The listing builds one solid part. Answer for the finished solid, in the listing's coordinates (mm). A direction names the side the tool comes from. Coordinates: 2 decimals unless noted, no trailing zeros. Order: outer loops, then holes, each group sorted by start corner. A loop starts at its lowest first (then second) coordinate and runs counter-clockwise, first axis right, second up. Notation, with made-up numbers: (30.25, -35.5) -> (58.25, -35.5) arc R17 ccw to (58.25, -7.5) -> close; hole circle Ø6 at (-40, 23.25). An arc over 180 degrees is marked (long way). Return JSON: item names as keys, results as strings.
from build123d import *

# Parameters (mm, degrees)
ENL_V_MAT_EXTRU_1_DEPTH = 149.219431924
ESQUISSE3_R             = 3.75
ENL_V_MAT_EXTRU_2_DEPTH = 131.858702424
ENL_V_MAT_EXTRU_3_DEPTH = 126.862394907
ENL_V_MAT_EXTRU_4_DEPTH = 10
CONG_1_R                = 1


with BuildPart() as part:
    # Esquisse1 → Révolution1 (revolve)
    with BuildSketch(Plane.XY, mode=Mode.PRIVATE) as r_volution1_sk:
        with BuildLine():
            Line((0, 0), (24.566275292, 0))
            Line((24.566275292, 0), (24.566275292, 25))
            Line((24.566275292, 25), (7.566275292, 25))
            ThreePointArc((7.566275292, 25), (6.152061729, 25.585786438), (5.566275292, 27))
            Line((5.566275292, 27), (5.566275292, 40))
            Line((5.566275292, 40), (-22.933724708, 40))
            Line((-22.933724708, 40), (-25.433724708, 37.5))
            Line((-25.433724708, 37.5), (-62.433724708, 37.5))
            Line((-62.433724708, 37.5), (-64.933724708, 40))
            Line((-64.933724708, 40), (-93.433724708, 40))
            Line((-93.433724708, 40), (-93.433724708, 27))
            ThreePointArc((-93.433724708, 27), (-94.019511146, 25.585786438), (-95.433724708, 25))
            Line((-95.433724708, 25), (-112.433724708, 25))
            Line((-112.433724708, 25), (-112.433724708, 0))
            Line((-112.433724708, 0), (0, 0))
        make_face()
    revolve(r_volution1_sk.sketch.rotate(Axis((-130.768922499, 0, 0), (1, 0, 0)), 90), axis=Axis((-130.768922499, 0, 0), (1, 0, 0)))

    # Esquisse2 → Enlèv. mat.-Extru.1 (cut, through all)
    with BuildSketch(Plane.ZY.offset(112.433724708)):
        with BuildLine():
            Line((0, 7), (0, 0))
            Line((0, 0), (43.449782835, 0))
            Line((43.449782835, 0), (43.449782835, 44.497429883))
            Line((43.449782835, 44.497429883), (0, 44.497429883))
            Line((0, 44.497429883), (0, 13))
            ThreePointArc((0, 13), (3, 10), (0, 7))
        make_face()
        with BuildLine():
            Line((-12, 7), (0, 7))
            ThreePointArc((0, 7), (3, 10), (0, 13))
            Line((0, 13), (-12, 13))
            ThreePointArc((-12, 13), (-15, 10), (-12, 7))
        make_face()
    extrude(amount=-ENL_V_MAT_EXTRU_1_DEPTH, mode=Mode.SUBTRACT)

    # Esquisse3 → Enlèv. mat.-Extru.2 (cut, through all)
    with BuildSketch(Plane.ZY.offset(93.433724708)):
        with Locations((-8.282209443, 30.909626441)):
            Circle(ESQUISSE3_R)
        with Locations((-22.627416998, 22.627416998)):
            Circle(ESQUISSE3_R)
        with Locations((-30.909626441, 8.282209443)):
            Circle(ESQUISSE3_R)
        with Locations((-30.909626441, -8.282209443)):
            Circle(ESQUISSE3_R)
        with Locations((-22.627416998, -22.627416998)):
            Circle(ESQUISSE3_R)
        with Locations((-8.282209443, -30.909626441)):
            Circle(ESQUISSE3_R)
        with Locations((8.282209443, -30.909626441)):
            Circle(ESQUISSE3_R)
        with Locations((22.627416998, -22.627416998)):
            Circle(ESQUISSE3_R)
        with Locations((30.909626441, -8.282209443)):
            Circle(ESQUISSE3_R)
    extrude(amount=-ENL_V_MAT_EXTRU_2_DEPTH, mode=Mode.SUBTRACT)

    # Esquisse4 → Enlèv. mat.-Extru.3 (cut, through all)
    with BuildSketch(Plane(origin=(0, 0, 0), x_dir=(1, 0, 0), z_dir=(0, 1, 0))):
        with BuildLine():
            Line((5.566275292, -31.140154495), (24.566275292, -40))
            Line((24.566275292, -40), (21.921370581, -25))
            Line((21.921370581, -25), (7.566275292, -25))
            ThreePointArc((7.566275292, -25), (6.152061729, -25.585786438), (5.566275292, -27))
            Line((5.566275292, -27), (5.566275292, -31.140154495))
        make_face()
        with BuildLine():
            Line((-5.433724708, -40), (5.566275292, -40))
            Line((5.566275292, -40), (5.566275292, -31.140154495))
            Line((5.566275292, -31.140154495), (-2.622958319, -27.321452148))
            ThreePointArc((-2.622958319, -27.321452148), (-4.722604922, -33.506811582), (-5.433724708, -40))
        make_face()
        with BuildLine():
            Line((-2.622958319, -27.321452148), (5.566275292, -31.140154495))
            Line((5.566275292, -31.140154495), (5.566275292, -27))
            ThreePointArc((5.566275292, -27), (6.152061729, -25.585786438), (7.566275292, -25))
            Line((7.566275292, -25), (21.921370581, -25))
            Line((21.921370581, -25), (19.356829962, -10.45576741))
            ThreePointArc((19.356829962, -10.45576741), (6.303432421, -16.199399791), (-2.622958319, -27.321452148))
        make_face()
        Polygon((5.566275292, -40), (24.566275292, -40), (5.566275292, -31.140154495), align=None)
        with BuildLine():
            Line((-7.154497255, -25.208360839), (-2.622958319, -27.321452148))
            ThreePointArc((-2.622958319, -27.321452148), (6.303432421, -16.199399791), (19.356829962, -10.45576741))
            Line((19.356829962, -10.45576741), (18.488589073, -5.531728645))
            ThreePointArc((18.488589073, -5.531728645), (3.259625276, -12.23263309), (-7.154497255, -25.208360839))
        make_face()
        with BuildLine():
            Line((21.921370581, -25), (24.566275292, -25))
            Line((24.566275292, -25), (24.566275292, -10))
            ThreePointArc((24.566275292, -10), (21.951603009, -10.114159057), (19.356829962, -10.45576741))
            Line((19.356829962, -10.45576741), (21.921370581, -25))
        make_face()
        Polygon((21.921370581, -25), (24.566275292, -40), (24.566275292, -25), align=None)
    extrude(amount=-ENL_V_MAT_EXTRU_3_DEPTH, mode=Mode.SUBTRACT)

    # Esquisse5 → Enlèv. mat.-Extru.4 (cut)
    with BuildSketch(Plane.ZY.offset(112.433724708)):
        with BuildLine():
            Line((20.615528128, -4), (-4, -4))
            Line((-4, -4), (-4, 3))
            Line((-4, 3), (-20.784609691, 3))
            ThreePointArc((-20.784609691, 3), (-3.501020872, -20.706106656), (20.615528128, -4))
        make_face()
    extrude(amount=-ENL_V_MAT_EXTRU_4_DEPTH, mode=Mode.SUBTRACT)

    # Congé1
    cong_1_edges = [part.edges().sort_by_distance(p)[0] for p in [
        (-102.433724708, -20.706106656, -3.501020872),
        (-102.433724708, 3, -12.392304845),
        (-102.433724708, -0.5, -4),
        (-102.433724708, -4, 8.307764064),
    ]]
    fillet(cong_1_edges, radius=CONG_1_R)


solid = part.part
1. Consider line 1 (Y direction, x = -60, z = -11); line 2 (Y direction, x = -36, z = -33); line 3 (Z direction, x = -38.5, y = -23). Determine where each line is inside the solid, lowest interval first. Write a range as from..to.
Answer block:
{"line 1": "y = -35.85..-33.49, -28.33..7, 13..28.33, 33.49..35.85", "line 2": "y = -17.81..-11.4, -5.17..5.17, 11.4..17.81", "line 3": "z = -29.62..-26.36, -18.9..18.9, 26.36..29.62"}
2. For faces 1 (the face through (3.45, -14.73, 12.09)), 2 (the face through (-93.434, -21, -18)), 3 (the face through (-44.2, -27.4, -25.6)), determine the directions among +Z, -Z, +X, -X, +Y, -Y from which every point of the face is accessible in a straight line to the end or side of a thin tool.
Answer block:
{"face 1": "+Y, -Y", "face 2": "-X", "face 3": "none"}
3. The part is cut by section A-A on x = -74.5. Give the number of separate pieces and of enclosed holes in the cut face, and give its area (3 significant figures).
Answer block:
{"separate pieces": "1", "enclosed holes": "9", "area": "3,290 mm2"}
4. The part is cut by section B-B on x = -1. Give the vertices of the cut face in (y, z).
Answer block:
{"outline": "(-36.62, 16.1) arc R40 ccw (long way) to (40, 0) -> (13, 0) -> (13, -12) arc R3 cw to (7, -12) -> (7, 0) -> (0, 0) -> (0, 16.1) -> close; hole circle Ø7.5 at (-30.91, -8.28); hole circle Ø7.5 at (-30.91, 8.28); hole circle Ø7.5 at (-22.63, -22.63); hole circle Ø7.5 at (-8.28, -30.91); hole circle Ø7.5 at (8.28, -30.91); hole circle Ø7.5 at (22.63, -22.63); hole circle Ø7.5 at (30.91, -8.28)"}
5. Determine the mould class of faces 4 (the face through (-62.59, -27.491, -25.734)), 5 (the face through (-108, -4, 8)), 6 (the face through (24.566, -6, -7)) for opening direction Y: pulls with the +Y half, pulls with the -Y half, needs draft (parallel to the pull), parting line crosses it, or undercut.
Answer block:
{"face 4": "parting line crosses it", "face 5": "undercut", "face 6": "needs draft"}
6. Each of these flat-tipped pins is pushed along its axis until it touches: pin 1 Ø7 at (x, z) = (-107, -9) entering from -Y; pin 2 Ø4 at (x, z) = (-67, -4.5) entering from +Y; pin 3 Ø13 at (x, z) = (-33.5, -5.5) entering from +Y; pin 4 Ø12 at (y, z) = (15.5, 9) entering from -X. Where does it stop, or does it pass through?
Answer block:
{"pin 1": "stops at y = -24.39", "pin 2": "stops at y = 39.92", "pin 3": "stops at y = 37.5", "pin 4": "passes through"}
